Check sheet for the modelled part. Datum: model origin and axes. Units: mm. Face numbers are marked on the shaded views. Give positions to 0.01 mm unless a question says otherwise; leave off trailing zeros. Order: outer loops, then holes, each group sorted by start corner. A loop starts at its lowest first (then second) coordinate and runs counter-clockwise, first axis right, second up.
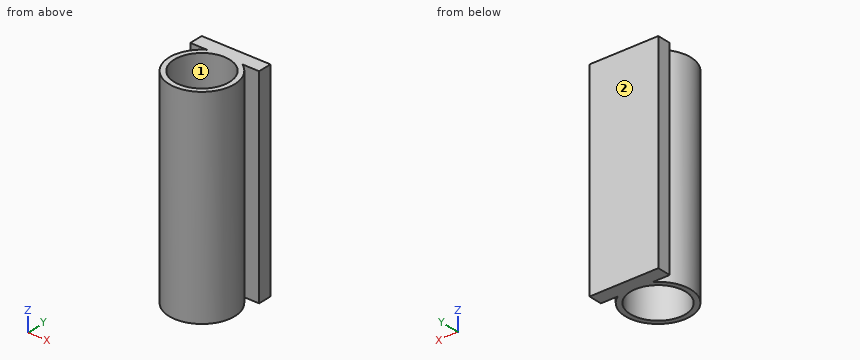
Autodesk Fusion 360 part; units mm, degrees
sketch "Sketch1" plane through (0, 0, 0) normal (0, 0, 1) x (1, 0, 0)
  circle A0 centre (0, 0) radius 8
  circle A1 centre (0, 0) radius 9.5
  line L0 (-10, 8) -> (10, 8)
  line L1 (10, 8) -> (10, 12)
  line L2 (10, 12) -> (-10, 12)
  line L3 (-10, 12) -> (-10, 8)
  dimension "d1" = 16
  dimension "d2" = 19
  dimension "d3" = 20
extrude "Extrude1" add sketch "Sketch1" along normal blind 60
1) Draft check along X on the marked faces 1 and 2. Enter one of: +X half, -X half, draft (parallel to the pull), parting line (faces both ways), or undercut.
Recorded:
face 1: undercut
face 2: draft
2) Section check C-C, the plane z = 28. Record the cut outline in (x, y), then the cut area to 3 significant figures.
Recorded:
outline: (-10, 8) - (-5.12, 8) arc R9.5 ccw (long way) to (5.12, 8) - (10, 8) - (10, 12) - (-10, 12) - close; hole circle Ø16 at (0, 0)
area: 152 mm2
3) Section check D-D, the plane x = 6.5. Record the cut outline in (y, z).
Recorded:
outline: (-6.93, 0) - (-4.66, 0) - (-4.66, 60) - (-6.93, 60) - close; (4.66, 0) - (6.93, 0) - (6.93, 60) - (4.66, 60) - close; (8, 0) - (12, 0) - (12, 60) - (8, 60) - close
4) Section check A-A, the plane y = 0. Record the cut outline in (x, z).
Recorded:
outline: (-9.5, 0) - (-8, 0) - (-8, 60) - (-9.5, 60) - close; (8, 0) - (9.5, 0) - (9.5, 60) - (8, 60) - close
5) Material ranges on L1, parallel to X at y = 0, z = 36; L2, parallel to Y at x = -5.5, z = 40; L3, parallel to Y at x = 8.75, z = 30, recorded low to high.
Recorded:
L1: x = -9.5 to -8, 8 to 9.5
L2: y = -7.75 to -5.81, 5.81 to 7.75, 8 to 12
L3: y = -3.7 to 3.7, 8 to 12
6) Section check B-B, the plane x = 0. Record the cut outline in (y, z).
Recorded:
outline: (-9.5, 0) - (-8, 0) - (-8, 60) - (-9.5, 60) - close; (8, 0) - (12, 0) - (12, 60) - (8, 60) - close
7) Depth check by flat-ended pin: pin 1 Ø8 at (y, z) = (-2, 46) entering from +X; pin 2 Ø3 at (x, z) = (3.5, 25.5) entering from -Y; pin 3 Ø2 at (y, z) = (-3.5, 18) entering from -X. Enter the tip coordinate at first touch or a pass-through.
Recorded:
pin 1: stops at x = 9.5
pin 2: stops at y = -9.29
pin 3: stops at x = -9.17
